```python
from build123d import *

# Parameters (mm, degrees)
F1_DEPTH    = 40
F4_DEPTH    = 40
F7_D        = 4
F8_T1_DEPTH = 45.0963937419
F8_T3_DEPTH = 44.9054294597


# Not quite as in the source:
# - a fillet or chamfer that OpenCascade refuses, or shapes differently, is made with other operations: its cross-section is extruded or revolved along the edge and cut away or added


with BuildPart() as f1:
    # F0 (on Right) → F1 (new body)
    with BuildSketch(Plane.YZ):
        with BuildLine():
            ThreePointArc((-63.4816033854, -7.334386461), (-67.4816033854, -11.334386461), (-63.4816033854, -15.334386461))
            Line((-63.4816033854, -15.334386461), (11.5183966146, -15.334386461))
            ThreePointArc((11.5183966146, -15.334386461), (16.1842937846, -12.1314406057), (14.8723445539, -6.6261479006))
            Line((14.8723445539, -6.6261479006), (-36.2252883959, 41.3947367846))
            Line((-36.2252883959, 41.3947367846), (-40.2507597139, 36.9440392082))
            Line((-40.2507597139, 36.9440392082), (-2.4015535455, 1.3738520994))
            ThreePointArc((-2.4015535455, 1.3738520994), (-1.0896043148, -4.1314406057), (-5.7555014847, -7.334386461))
            Line((-5.7555014847, -7.334386461), (-63.4816033854, -7.334386461))
        make_face()
    extrude(amount=F1_DEPTH)

    # F3 (on offset) → F4 (join)
    with BuildSketch(Plane.YZ.offset(40)):
        with BuildLine():
            Line((14.8723445539, -6.6261479006), (-36.2252883959, 41.3947367846))
            Line((-36.2252883959, 41.3947367846), (-40.2507597139, 36.9440392082))
            Line((-40.2507597139, 36.9440392082), (-2.4015535455, 1.3738520994))
            ThreePointArc((-2.4015535455, 1.3738520994), (-1.0896043148, -4.1314406057), (-5.7555014847, -7.334386461))
            Line((-5.7555014847, -7.334386461), (-63.4816033854, -7.334386461))
            ThreePointArc((-63.4816033854, -7.334386461), (-67.4816033854, -11.334386461), (-63.4816033854, -15.334386461))
            Line((-63.4816033854, -15.334386461), (11.5183966146, -15.334386461))
            ThreePointArc((11.5183966146, -15.334386461), (16.1842937846, -12.1314406057), (14.8723445539, -6.6261479006))
        make_face()
        with BuildLine():
            Line((-40.2507597139, 36.9440392082), (-36.2252883959, 41.3947367846))
            Line((-36.2252883959, 41.3947367846), (-37.8997588755, 42.9683821605))
            ThreePointArc((-37.8997588755, 42.9683821605), (-37.8866027682, 42.7814716227), (-37.8822141892, 42.5941500472))
            ThreePointArc((-37.8822141892, 42.5941500472), (-39.0988744687, 39.7213430575), (-42.0087241892, 38.5961511452))
            Line((-42.0087241892, 38.5961511452), (-40.2507597139, 36.9440392082))
        make_face()
        with BuildLine():
            ThreePointArc((-37.8822141892, 42.5941500472), (-37.8866027682, 42.7814716227), (-37.8997588755, 42.9683821605))
            ThreePointArc((-37.8997588755, 42.9683821605), (-44.7970348661, 45.3334602563), (-42.0087241892, 38.5961511452))
            ThreePointArc((-42.0087241892, 38.5961511452), (-39.0988744687, 39.7213430575), (-37.8822141892, 42.5941500472))
        make_face()
    extrude(amount=F4_DEPTH)

    # F7 (through all)
    with Locations(Plane.YZ.offset(120)):
        with Locations((-41.8822141892, 42.5941500472)):
            Hole(F7_D / 2)

    # F8: fillet of radius 2 on 2 edges, made by hand

    # F8_s2 → F8_t1 (cut)
    with BuildSketch(Plane.YZ.offset(-5.0963937419)):
        with BuildLine():
            ThreePointArc((-37.592731539, 39.8828452812), (-36.190570233, 40.5396197416), (-34.7397810103, 39.9986764439))
            Line((-34.7397810103, 39.9986764439), (-36.2252883959, 41.3947367846))
            Line((-36.2252883959, 41.3947367846), (-37.592731539, 39.8828452812))
        make_face()
    extrude(amount=F8_T1_DEPTH, mode=Mode.SUBTRACT)

    # F8_s4 → F8_t3 (cut)
    with BuildSketch(Plane.YZ.offset(-4.9054294597)):
        with BuildLine():
            ThreePointArc((-38.9345553117, 38.3992794224), (-39.4496135236, 36.9765661286), (-38.8209149921, 35.6002899083))
            Line((-38.8209149921, 35.6002899083), (-40.2507597139, 36.9440392082))
            Line((-40.2507597139, 36.9440392082), (-38.9345553117, 38.3992794224))
        make_face()
    extrude(amount=F8_T3_DEPTH, mode=Mode.SUBTRACT)


solid = f1.part
```
The model under review builds one solid part; all positions refer to its coordinate system, in mm. A direction names the side the tool comes from. Round coordinates to 2 decimals unless told otherwise and drop trailing zeros. Loops run counter-clockwise (first coordinate to the right, second up) from the corner with the lowest first, then second, coordinate; pieces in that order, holes last. Notation, with made-up numbers: (-19, 25) - (23, 25) arc R7 cw to (23, 34) - close; hole circle Ø5 at (41.5, 29). An arc over 180 degrees is marked (long way). Write each question's results on one line, items separated by ' | '. Start each with the question number.
Q1. Take a section at D-D on x = 66. Give the boundary of the cut face in (y, z), plus the area to 3 significant figures.
Q2. Take a section at B-B on x = 30. Give the boundary of the cut face in (y, z).
Q3. Take a section at A-A on y = -33.5. Give the boundary of the cut face in (x, z).
Q4. Draft analysis for pull direction Z (two halves, no side actions). For faces 5 (the flat face through (80, -23, -9)), 6 (the cylindrical face through (39.44, -1.06, -4.05)), 7 (the cylindrical face through (39.44, -67.48, -11.25)), state which applies: pulls with the +Z half, pulls with the -Z half, needs draft (parallel to the pull), parting line crosses it, or undercut.
Q5. Take a section at C-C on y = -58. Give the boundary of the cut face in (x, z), plus the area to 3 significant figures.
Q6. Insertion check: P1, Ø10, axis at y = -10.5, z = 21.5, coming from the +X side; P2, Ø10, axis at x = 58.5, z = 31, coming from the -Y side; P3, Ø3.5, axis at y = -41.88, z = 42.59, coming from the +X side; P4, Ø1.5, axis at x = 61.5, y = 7.5, coming from the +Z side. Each pin has a flat end and moves straight along its axis. Give the tip position at first contact, or say it passes through.
Q7. Tool access review of faces 1 (the flat face through (39, -34, -7.334)), 2 (the cylindrical face through (19.72, -36.21, 40.54)), 3 (the cylindrical face through (59.72, -39.884, 42.682)), 4 (the cylindrical face through (19.72, -39.45, 37)): name each direction out of +Z, -Z, +X, -X, +Y, -Y from which nothing blocks a thin tool from reaching the whole face with its end or side.
Q8. Wall thickness on line 1 along Z through (x, y) = (10, -50.5); line 2 along Z through (x, y) = (13, -34); line 3 along Z through (x, y) = (64.5, -13): over which ranges is each line inside the solid? List them lowest first. Write a range as [from, to].
Data:
1) outline: (-63.48, -15.33) - (11.52, -15.33) arc R5 ccw to (14.87, -6.63) - (-37.9, 42.97) arc R4 ccw (long way) to (-42.01, 38.6) - (-2.4, 1.37) arc R5 cw to (-5.76, -7.33) - (-63.48, -7.33) arc R4 ccw to start; hole circle Ø4 at (-41.88, 42.59) | area: 1,150 mm²
2) outline: (-63.48, -15.33) - (11.52, -15.33) arc R5 ccw to (14.87, -6.63) - (-34.74, 40) arc R2 ccw to (-37.59, 39.88) - (-38.93, 38.4) arc R2 ccw to (-38.82, 35.6) - (-2.4, 1.37) arc R5 cw to (-5.76, -7.33) - (-63.48, -7.33) arc R4 ccw to start
3) outline: (0, -15.33) - (80, -15.33) - (80, -7.33) - (0, -7.33) - close; (0, 30.6) - (80, 30.6) - (80, 38.83) - (0, 38.83) - close
4) face 5: needs draft | face 6: undercut | face 7: parting line crosses it
5) outline: (0, -15.33) - (80, -15.33) - (80, -7.33) - (0, -7.33) - close | area: 640 mm²
6) P1: stops at x = 80 | P2: stops at y = -39.25 | P3: passes through | P4: stops at z = 1.01
7) face 1: +X, -X, -Y | face 2: +Z, -X | face 3: +X, -X | face 4: -X, -Y
8) line 1: z = [-15.33, -7.33] | line 2: z = [-15.33, -7.33], [31.07, 39.3] | line 3: z = [-15.33, -7.33], [11.33, 19.57]
